```python
from build123d import *

# Parameters (mm, degrees)
F0_W     = 350
F0_H     = 200
F1_DEPTH = 6
F2_SIZE  = 5.99999
F3_DEPTH = 3


# Not quite as in the source:
# - a fillet or chamfer is up to 0.001 mm smaller than in the source, because OpenCascade refuses the exact size


with BuildPart() as f1:
    # F0 (on Top) → F1 (new body)
    with BuildSketch(Plane.XY):
        with Locations((103.189206589, -5.372708199)):
            Rectangle(F0_W, F0_H)
    extrude(amount=F1_DEPTH)

    # F2 (size 6 in the source; OpenCascade refuses exactly that, so slightly less here)
    f2_edges = [f1.edges().sort_by_distance(p)[0] for p in [
        (103.189207, -105.372708, 6),
    ]]
    chamfer(f2_edges, length=F2_SIZE)

    # F3 (cut): a face of the model
    f3_faces = [f1.faces().sort_by_distance(p)[0] for p in [
        (103.189206589, 94.627291801, 3),
    ]]
    extrude(f3_faces, amount=-F3_DEPTH, mode=Mode.SUBTRACT)


solid = f1.part
```
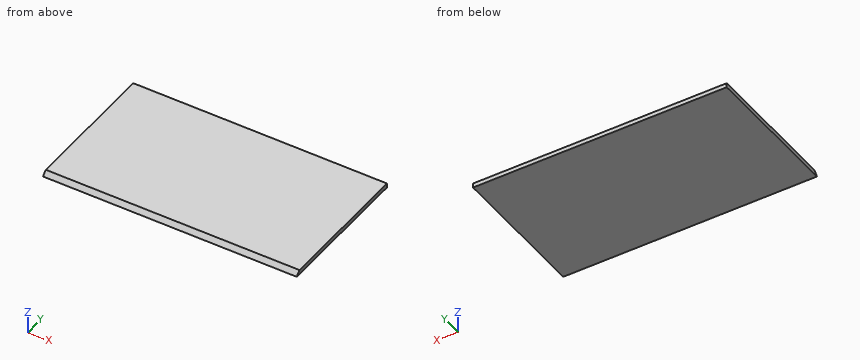
Design review of the part built by this model. Coordinates are the model's own, in mm. Coordinates: 2 decimals unless noted, no trailing zeros. Order: outer loops, then holes, each group sorted by start corner. A loop starts at its lowest first (then second) coordinate and runs counter-clockwise, first axis right, second up. Notation, with made-up numbers: (36, 49.25) -> (75, 49.25) arc R32 cw to (75, 84.25) -> close; hole circle Ø8 at (60, 76.25). An arc over 180 degrees is marked (long way). One line per item, written item: value. Start each with the question number.
Q1. Take a section at B-B, the plane z = 4.5. State the section outline as (x, y) points.
Q2. Insertion check: pin 1 Ø1 at (x, z) = (146, 4.5) entering from -Y; pin 2 Ø8 at (x, y) = (217.5, 20) entering from -Z. Each pin has a flat end and moves straight along its axis. Give the tip position at first contact, or say it passes through.
Q3. For probe 1 along Y at (x, z) = (-9.5, 4); probe 2 along Y at (x, z) = (230, 2), list the stretches that pass through material, from the lowest coordinate up.
Values follow:
1. outline: (-71.81, -100.87) -> (278.19, -100.87) -> (278.19, 91.63) -> (-71.81, 91.63) -> close
2. pin 1: stops at y = -101.37
2. pin 2: stops at z = 0
3. probe 1: y = -101.37 to 91.63
3. probe 2: y = -103.37 to 91.63
